Check sheet for the drawn part. Datum: minimum x, y, z corner. Units: mm. Round coordinates to 2 decimals unless told otherwise and drop trailing zeros. Write each loop counter-clockwise with the first axis right and the second up, starting at its lowest first coordinate (ties: lowest second). Pieces come first, ordered by that corner, then holes. Notation, with made-up numbers: M 19.5,51.25 L 69.5,51.25 A23 ccw 69.5,70.25 Z; hole C 66.25,17.5 d7. An arc over 180 degrees is marked long. One line per item, written item: value.
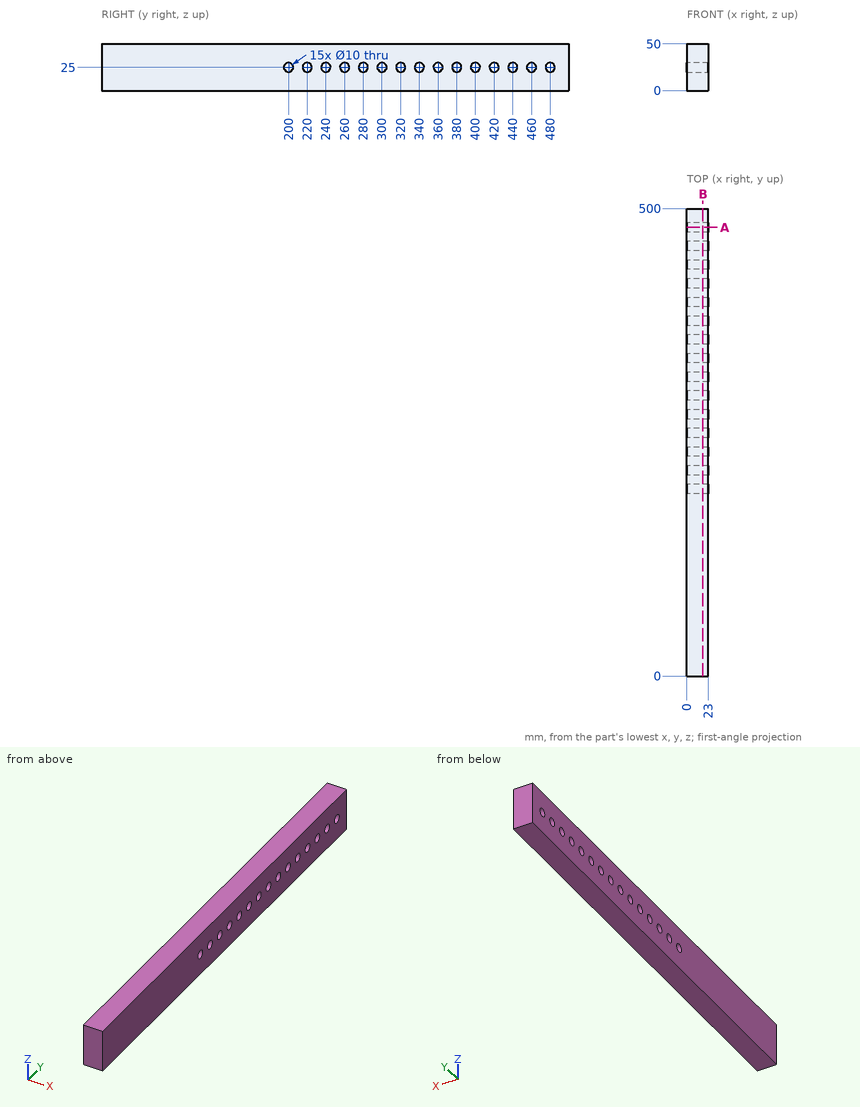
Q1. Sectioned sample at B-B on x = 17. State how many separate pieces and enclosed holes the cut face has, and give its area (3 significant figures).
Completed:
separate pieces: 1
enclosed holes: 15
area: 23,800 mm^2
Q2. Depth check by flat-ended pin: P1, Ø6, axis at y = 440, z = 25, coming from the +X side. Enter the tip coordinate at first touch or a pass-through.
Completed:
P1: through
Q3. Scan lines: line 1 (Z direction, x = 9.5, y = 340); line 2 (Z direction, x = 10.75, y = 281.5). Record each from-to range of solid material in increasing order. Write a range as [from, to].
Completed:
line 1: [0, 20], [30, 50]
line 2: [0, 20.23], [29.77, 50]
Q4. Sectioned sample at A-A on y = 480. Enter the section's corners in (x, z).
Completed:
outline: M 0,0 L 23,0 L 23,20 L 0,20 Z; M 0,30 L 23,30 L 23,50 L 0,50 Z
